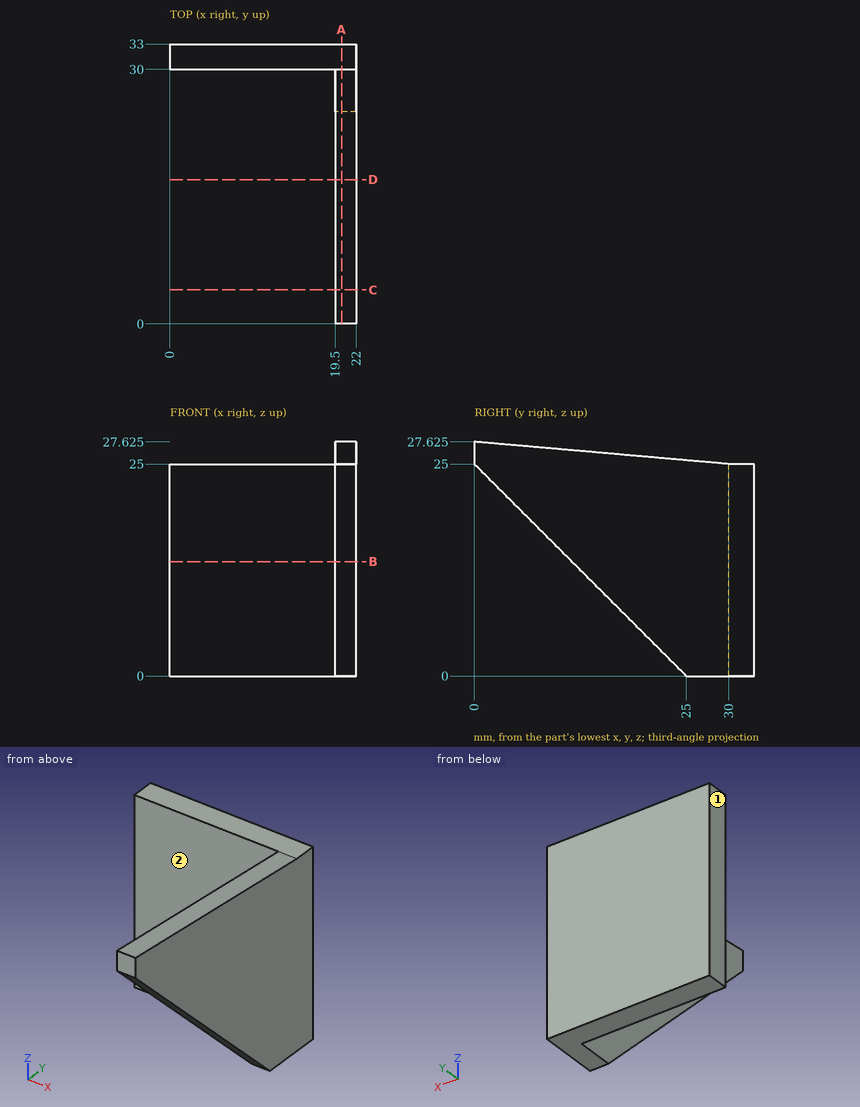
Input: dimensioned drawing with shaded views. Units: mm. Origin: part minimum x, y, z. A direction names the side the tool comes from. Coordinates: 2 decimals unless noted, no trailing zeros. Loops run counter-clockwise (first coordinate to the right, second up) from the corner with the lowest first, then second, coordinate; pieces in that order, holes last. Notation, with made-up numbers: M 50.25,68 L 107.25,68 A11 cw 107.25,79 Z; hole C 85.5,19.5 d2. An arc over 180 degrees is marked long. Use a Markdown table: item, result. Add a question column.
1) Pin query (flat end, axial travel): P1, Ø6, axis at x = 17.5, z = 16.5, coming from the -Y side (1 decimal); P2, Ø10, axis at x = 12.5, z = 12, coming from the -Y side; P3, Ø5, axis at y = 16.5, z = 13.5, coming from the -X side. Return the tip coordinate at first contact, or that it passes through.
2) Section C-C, the plane y = 4. Return the cut outline in (x, z) (1 decimal), plus the area to 3 significant figures.
3) Set-up query: the marked faces 1 and 2. Return all of +Z, -Z, +X, -X, +Y, -Y with unobstructed straight access to the full face (end or side cutting, diameter ignored); none if empty.
4) Section A-A, the plane x = 20.25. Return the cut outline in (y, z) (1 decimal), plus the area to 3 significant figures.
5) Line query: L1, parallel to Y at x = 6.75, z = 17.75; L2, parallel to X at y = 27.5, z = 20.75; L3, parallel to Z at x = 12.5, y = 30.5. Output: solid intervals per line, ascending. Write a range as from..to.
6) Section D-D, the plane y = 17. Return the cut outline in (x, z).
7) Section B-B, the plane z = 13.5. Return the cut outline in (x, y).
Answer below:
| question | item | result |
|---|---|---|
| 1 | P1 | y = 6.3 |
| 1 | P2 | y = 30 |
| 1 | P3 | x = 19.5 |
| 2 | outline | M 19.5,21 L 22,21 L 22,27.3 L 19.5,27.3 Z |
| 2 | area | 15.7 mm2 |
| 3 | face 1 | +Z, -Z, -X, +Y, -Y |
| 3 | face 2 | +Z, -Z, -X, -Y |
| 4 | outline | M 0,25 L 25,0 L 33,0 L 33,25 L 30,25 L 0,27.6 Z |
| 4 | area | 552 mm2 |
| 5 | L1 | 30..33 |
| 5 | L2 | 19.5..22 |
| 5 | L3 | 0..25 |
| 6 | outline | M 19.5,8 L 22,8 L 22,26.14 L 19.5,26.14 Z |
| 7 | outline | M 0,30 L 19.5,30 L 19.5,11.5 L 22,11.5 L 22,33 L 0,33 Z |
